Design review of the part built by this model. Coordinates are the model's own, in mm. Give positions to 0.01 mm unless a question says otherwise; leave off trailing zeros. Loops run counter-clockwise (first coordinate to the right, second up) from the corner with the lowest first, then second, coordinate; pieces in that order, holes last. Notation, with made-up numbers: M 31.25,65 L 79.25,65 A5 cw 79.25,71 Z; hole C -18,-4.75 d7. An arc over 180 degrees is marked long. Answer as CSV lines item,"result".
```python
from build123d import *

# Parameters (mm, degrees)
F0_W     = 88.65
F0_H     = 38.5064
F0_R     = 1.905
F0_R_2   = 2.5
F1_DEPTH = 6.2484


with BuildPart() as f1:
    # F0 (on Front) → F1 (new body)
    with BuildSketch(Plane.XZ):
        with Locations((4.548196, -2.739448)):
            Rectangle(F0_W, F0_H)
        with Locations((-19.776804, -15.795048)):
            Circle(F0_R, mode=Mode.SUBTRACT)
        with Locations((-19.776804, -2.739448)):
            Circle(F0_R, mode=Mode.SUBTRACT)
        with Locations((3.395596, -2.739448)):
            Circle(F0_R_2, mode=Mode.SUBTRACT)
        with Locations((-19.776804, 10.316152)):
            Circle(F0_R, mode=Mode.SUBTRACT)
        with Locations((9.389996, -2.739448)):
            Circle(F0_R_2, mode=Mode.SUBTRACT)
        with Locations((15.384396, -2.739448)):
            Circle(F0_R_2, mode=Mode.SUBTRACT)
        with Locations((21.378796, -2.739448)):
            Circle(F0_R_2, mode=Mode.SUBTRACT)
        with Locations((27.373196, -2.739448)):
            Circle(F0_R_2, mode=Mode.SUBTRACT)
        with Locations((33.373196, -2.739448)):
            Circle(F0_R_2, mode=Mode.SUBTRACT)
        with Locations((39.373196, -2.739448)):
            Circle(F0_R_2, mode=Mode.SUBTRACT)
    extrude(amount=-F1_DEPTH)


solid = f1.part
```
1. We need section C-C, the plane x = 2.5. Write out the cut boundary in (y, z).
Answer block:
outline,"M 0,-21.99 L 6.25,-21.99 L 6.25,-5.07 L 0,-5.07 Z; M 0,-0.41 L 6.25,-0.41 L 6.25,16.51 L 0,16.51 Z"
2. We need section B-B, the plane y = 1. Count the separate pieces of the cut face and the enclosed holes in it, plus the area to 3 significant figures.
Answer block:
separate pieces,"1"
enclosed holes,"10"
area,"3,240 mm²"
3. We need section A-A, the plane x = 40.5. Write out the cut boundary in (y, z).
Answer block:
outline,"M 0,-21.99 L 6.25,-21.99 L 6.25,-4.97 L 0,-4.97 Z; M 0,-0.51 L 6.25,-0.51 L 6.25,16.51 L 0,16.51 Z"
4. To check wall thickness, follow L1, parallel to Z at x = -20, y = 3; L2, parallel to X at y = 4, z = 10; L3, parallel to X at y = 1.75, z = -17.5. State the ranges of each line that lie inside material, in increasing order. Write a range as [from, to].
Answer block:
L1,"[-21.99, -17.69], [-13.9, -4.63], [-0.85, 8.42], [12.21, 16.51]"
L2,"[-39.78, -21.66], [-17.9, 48.87]"
L3,"[-39.78, -20.63], [-18.93, 48.87]"
5. The part is to be moulded in two halves that separate along X. For faces 1 (the flat face through (4, 0, 2)), 2 (the cylindrical face through (24.876, 3.08, -2.63)), 3 (the flat face through (48.873, 3, -3)), say which applies: pulls with the +X half, pulls with the -X half, needs draft (parallel to the pull), parting line crosses it, or undercut.
Answer block:
face 1,"needs draft"
face 2,"undercut"
face 3,"pulls with the +X half"
